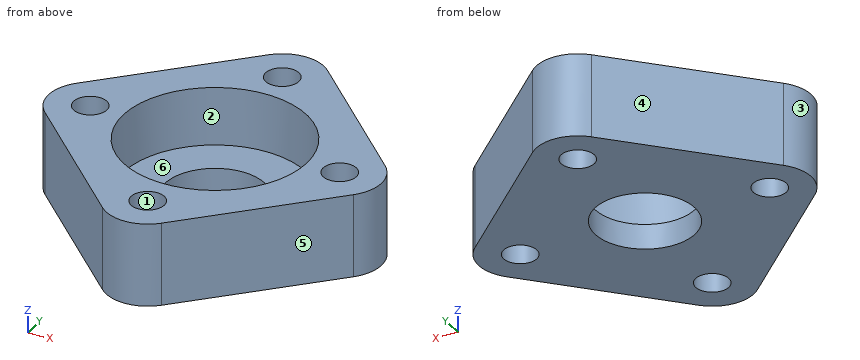
```python
from build123d import *

# Parameters (mm, degrees)
SKETCH1_R           = 2
BOSS_EXTRUDE1_DEPTH = 10
SKETCH2_R           = 11
CUT_EXTRUDE1_DEPTH  = 7
SKETCH3_R           = 6
CUT_EXTRUDE2_DEPTH  = 7


with BuildPart() as part:
    # Sketch1 → Boss-Extrude1 (new body)
    with BuildSketch(Plane.XY):
        with BuildLine():
            Line((-18.535533906, 3.535533906), (-3.535533906, 18.535533906))
            ThreePointArc((-3.535533906, 18.535533906), (0, 20), (3.535533906, 18.535533906))
            Line((3.535533906, 18.535533906), (18.535533906, 3.535533906))
            ThreePointArc((18.535533906, 3.535533906), (20, 0), (18.535533906, -3.535533906))
            Line((18.535533906, -3.535533906), (3.535533906, -18.535533906))
            ThreePointArc((3.535533906, -18.535533906), (0, -20), (-3.535533906, -18.535533906))
            Line((-3.535533906, -18.535533906), (-18.535533906, -3.535533906))
            ThreePointArc((-18.535533906, -3.535533906), (-20, 0), (-18.535533906, 3.535533906))
        make_face()
        with Locations((0, 15)):
            Circle(SKETCH1_R, mode=Mode.SUBTRACT)
        with Locations((15, 0)):
            Circle(SKETCH1_R, mode=Mode.SUBTRACT)
        with Locations((0, -15)):
            Circle(SKETCH1_R, mode=Mode.SUBTRACT)
        with Locations((-15, 0)):
            Circle(SKETCH1_R, mode=Mode.SUBTRACT)
    extrude(amount=BOSS_EXTRUDE1_DEPTH)

    # Sketch2 → Cut-Extrude1 (cut)
    with BuildSketch(Plane.XY.offset(10)):
        Circle(SKETCH2_R)
    extrude(amount=-CUT_EXTRUDE1_DEPTH, mode=Mode.SUBTRACT)

    # Sketch3 → Cut-Extrude2 (cut)
    with BuildSketch(Plane.XY.offset(3)):
        Circle(SKETCH3_R)
    extrude(amount=-CUT_EXTRUDE2_DEPTH, mode=Mode.SUBTRACT)


solid = part.part
```
Model file for the job. Use its own axes, mm. Face numbers are marked on the shaded views. A direction names the side the tool comes from. Coordinates: 2 decimals unless noted, no trailing zeros. Write each loop counter-clockwise with the first axis right and the second up, starting at its lowest first coordinate (ties: lowest second). Pieces come first, ordered by that corner, then holes. Notation, with made-up numbers: (-39, 42.5) - (18, 42.5) arc R17 ccw to (18, 60.5) - close; hole circle Ø11 at (35.25, 4.5). An arc over 180 degrees is marked (long way). One line per item, written item: value. Start each with the question number.
1. Slice it at B-B (y = 15). Write the cut outline in (x, z), plus the area to 3 significant figures.
2. Probe line 1 (Y direction, x = 0, z = 1.05); line 2 (X direction, y = -0.5, z = 9.25); line 3 (X direction, y = -0.5, z = 1). List the from-to ranges inside material, lowest first. Write a range as from..to.
3. Mould opens along Y. For the marked faces 1, 2, 3 and 4 say: released by +Y, released by -Y, zero draft, split by the parting line, or undercut.
4. Slice it at D-D (x = 16). Write the cut outline in (y, z), plus the area to 3 significant figures.
5. Slice it at A-A (x = 0). Write the cut outline in (y, z).
6. Slice it at C-C (z = 2). Write the cut outline in (x, y), plus the area to 3 significant figures.
7. Flat gauge pins, fed straight in: pin 1 (5 mm diameter, centred on y = 15.5, z = 2.5, fed in from +X); pin 2 (4.5 mm diameter, centred on x = 0, y = -15, fed in from -Z); pin 3 (3 mm diameter, centred on y = -7.5, z = 7.5, fed in from -X); pin 4 (6 mm diameter, centred on y = -10.5, z = 8.5, fed in from +X). Where does each tip first touch, or does it go through?
8. Tool access for the marked faces 5 and 6: list every direction of +Z, -Z, +X, -X, +Y, -Y with a clear straight run to the whole face (end or side of a thin tool).
Answers below:
1. outline: (-7.07, 0) - (-2, 0) - (-2, 10) - (-7.07, 10) - close; (2, 0) - (7.07, 0) - (7.07, 10) - (2, 10) - close
1. area: 101 mm^2
2. line 1: y = -20..-17, -13..-6, 6..13, 17..20
2. line 2: x = -19.97..-16.94, -13.06..-10.99, 10.99..13.06, 16.94..19.97
2. line 3: x = -19.97..-16.94, -13.06..-5.98, 5.98..13.06, 16.94..19.97
3. face 1: undercut
3. face 2: undercut
3. face 3: split by the parting line
3. face 4: released by +Y
4. outline: (-6.07, 0) - (-1.73, 0) - (-1.73, 10) - (-6.07, 10) - close; (1.73, 0) - (6.07, 0) - (6.07, 10) - (1.73, 10) - close
4. area: 86.8 mm^2
5. outline: (-20, 0) - (-17, 0) - (-17, 10) - (-20, 10) - close; (-13, 0) - (-6, 0) - (-6, 3) - (-11, 3) - (-11, 10) - (-13, 10) - close; (6, 0) - (13, 0) - (13, 10) - (11, 10) - (11, 3) - (6, 3) - close; (17, 0) - (20, 0) - (20, 10) - (17, 10) - close
6. outline: (-18.54, -3.54) - (-3.54, -18.54) arc R5 ccw to (3.54, -18.54) - (18.54, -3.54) arc R5 ccw to (18.54, 3.54) - (3.54, 18.54) arc R5 ccw to (-3.54, 18.54) - (-18.54, 3.54) arc R5 ccw to start; hole circle Ø4 at (-15, 0); hole circle Ø12 at (0, 0); hole circle Ø4 at (0, -15); hole circle Ø4 at (0, 15); hole circle Ø4 at (15, 0)
6. area: 789 mm^2
7. pin 1: stops at x = 9.07
7. pin 2: stops at z = 0
7. pin 3: stops at x = -16.07
7. pin 4: stops at x = 14.57
8. face 5: +Z, -Z, +X, -Y
8. face 6: +Z
